Check sheet for the modelled part. Datum: model origin and axes. Units: mm. Round coordinates to 2 decimals unless told otherwise and drop trailing zeros. Loops run counter-clockwise (first coordinate to the right, second up) from the corner with the lowest first, then second, coordinate; pieces in that order, holes last. Notation, with made-up numbers: (74.5, 47.25) - (98.5, 47.25) arc R19 cw to (98.5, 54.25) - close; hole circle Ø1 at (64, 86.5). An arc over 180 degrees is marked (long way). Put each result on its own line as item: value.
```python
from build123d import *

# Parameters (mm, degrees)
F0_W     = 7.62
F0_H     = 114.3
F1_DEPTH = 3.81
F2_W     = 38.1
F2_H     = 38.1
F2_W_2   = 7.62
F2_H_2   = 7.62
F3_DEPTH = 5.08


with BuildPart() as f1:
    # F0 (on Front) → F1 (new body, symmetric)
    with BuildSketch(Plane.XZ):
        Rectangle(F0_W, F0_H)
        with BuildLine():
            Line((-3.81, 57.15), (3.81, 57.15))
            Line((3.81, 57.15), (13.606083, 68.824517))
            Line((13.606083, 68.824517), (8.526083, 68.824517))
            ThreePointArc((8.526083, 68.824517), (0, 62.23), (-8.526083, 68.824517))
            Line((-8.526083, 68.824517), (-13.606083, 68.824517))
            Line((-13.606083, 68.824517), (-3.81, 57.15))
        make_face()
    extrude(amount=F1_DEPTH, both=True)

    # F2 (on face) → F3 (join)
    with BuildSketch(Plane(origin=(0, 0, -57.15), x_dir=(1, 0, 0), z_dir=(0, 0, -1))):
        Rectangle(F2_W, F2_H)
        Rectangle(F2_W_2, F2_H_2, mode=Mode.SUBTRACT)
    extrude(amount=-F3_DEPTH)


solid = f1.part
```
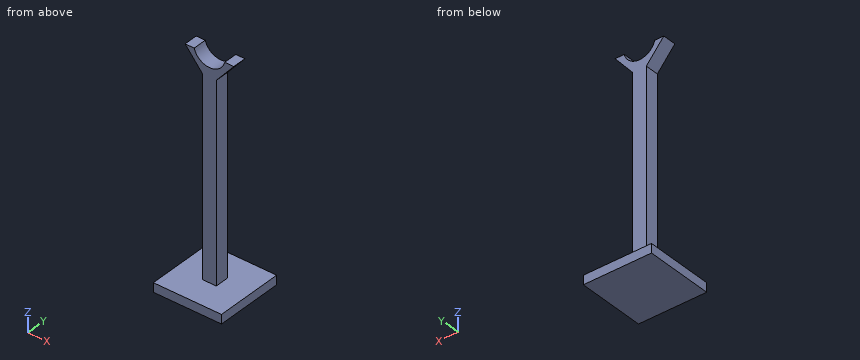
Item 1: Section check B-B on x = 0. Enter the section's corners in (y, z), then the cut area to 3 significant figures.
Filled sheet:
outline: (-19.05, -57.15) - (19.05, -57.15) - (19.05, -52.07) - (3.81, -52.07) - (3.81, 62.23) - (-3.81, 62.23) - (-3.81, -52.07) - (-19.05, -52.07) - close
area: 1,060 mm²
Item 2: Section check A-A on x = -7. Enter the section's corners in (y, z).
Filled sheet:
outline: (-19.05, -57.15) - (19.05, -57.15) - (19.05, -52.07) - (-19.05, -52.07) - close; (-3.81, 60.95) - (3.81, 60.95) - (3.81, 65.69) - (-3.81, 65.69) - close
Item 3: Thickness scan on line 1 (Z direction, x = 0.5, y = -5); line 2 (Z direction, x = 4, y = -2); line 3 (X direction, y = 3, z = 15). Record the ranges inside material, lowest first. Write a range as from..to.
Filled sheet:
line 1: -57.15..-52.07
line 2: -57.15..-52.07, 57.38..63.19
line 3: -3.81..3.81
Item 4: Go/stop test with flat-tipped pins: pin 1 (6 mm diameter, centred on y = 2.5, z = -27.5, fed in from -X); pin 2 (4 mm diameter, centred on y = -0.5, z = 12, fed in from +X); pin 3 (22 mm diameter, centred on x = 6, z = -4, fed in from +Y); pin 4 (4 mm diameter, centred on y = 6.5, z = -30, fed in from -X). Record where each tip stops, or that it passes through.
Filled sheet:
pin 1: x = -3.81
pin 2: x = 3.81
pin 3: y = 3.81
pin 4: through
Item 5: Section check C-C on z = 0.5. Enter the section's corners in (x, y), then the cut area to 3 significant figures.
Filled sheet:
outline: (-3.81, -3.81) - (3.81, -3.81) - (3.81, 3.81) - (-3.81, 3.81) - close
area: 58.1 mm²
Item 6: Section check D-D on y = 10.5. Enter the section's corners in (x, z).
Filled sheet:
outline: (-19.05, -57.15) - (19.05, -57.15) - (19.05, -52.07) - (-19.05, -52.07) - close
